```python
from build123d import *

# Parameters (mm, degrees)
SKETCH_1_R          = 13
EXTRUDE_1_DEPTH     = 4
SKETCH_2_R          = 6
CUT_EXTRUDE_1_DEPTH = 4
CUT_EXTRUDE_START   = -0.8
SKETCH_3_R          = 13
SKETCH_3_R_2        = 12
CUT_EXTRUDE_2_DEPTH = 0.4
CUT_EXTRUDE_START_2 = -3.2
SKETCH_3_3_R        = 13
SKETCH_3_3_R_2      = 12
CUT_EXTRUDE_3_DEPTH = 0.4


with BuildPart() as part:
    # Sketch 1 → Extrude 1 (new body)
    with BuildSketch(Plane(origin=(0, 0, 0), x_dir=(1, 0, 0), z_dir=(0, 1, 0))):
        Circle(SKETCH_1_R)
    extrude(amount=EXTRUDE_1_DEPTH)

    # Sketch 2 → Cut-Extrude 1 (cut)
    with BuildSketch(Plane.XZ):
        Circle(SKETCH_2_R)
    extrude(amount=-CUT_EXTRUDE_1_DEPTH, mode=Mode.SUBTRACT)

    # Sketch 3 → Cut-Extrude 2 (cut)
    with BuildSketch(Plane.XZ.offset(CUT_EXTRUDE_START)):
        Circle(SKETCH_3_R)
        Circle(SKETCH_3_R_2, mode=Mode.SUBTRACT)
    extrude(amount=-CUT_EXTRUDE_2_DEPTH, mode=Mode.SUBTRACT)

    # Sketch 3_3 → Cut-Extrude 3 (cut)
    with BuildSketch(Plane.XZ.offset(CUT_EXTRUDE_START_2)):
        Circle(SKETCH_3_3_R)
        Circle(SKETCH_3_3_R_2, mode=Mode.SUBTRACT)
    extrude(amount=CUT_EXTRUDE_3_DEPTH, mode=Mode.SUBTRACT)


solid = part.part
```
The model under review builds one solid part; all positions refer to its coordinate system, in mm. A direction names the side the tool comes from. Round coordinates to 2 decimals unless told otherwise and drop trailing zeros. Loops run counter-clockwise (first coordinate to the right, second up) from the corner with the lowest first, then second, coordinate; pieces in that order, holes last.
Item 1: Take a section at B-B (x = 0). Write out the cut boundary in (y, z), then the cut area to 3 significant figures.
Determined:
outline: (0, -13) - (0.8, -13) - (0.8, -12) - (1.2, -12) - (1.2, -13) - (2.8, -13) - (2.8, -12) - (3.2, -12) - (3.2, -13) - (4, -13) - (4, -6) - (0, -6) - close; (0, 6) - (4, 6) - (4, 13) - (3.2, 13) - (3.2, 12) - (2.8, 12) - (2.8, 13) - (1.2, 13) - (1.2, 12) - (0.8, 12) - (0.8, 13) - (0, 13) - close
area: 54.4 mm2
Item 2: Take a section at A-A (z = 0). Write out the cut boundary in (x, y).
Determined:
outline: (-13, 0) - (-6, 0) - (-6, 4) - (-13, 4) - (-13, 3.2) - (-12, 3.2) - (-12, 2.8) - (-13, 2.8) - (-13, 1.2) - (-12, 1.2) - (-12, 0.8) - (-13, 0.8) - close; (6, 0) - (13, 0) - (13, 0.8) - (12, 0.8) - (12, 1.2) - (13, 1.2) - (13, 2.8) - (12, 2.8) - (12, 3.2) - (13, 3.2) - (13, 4) - (6, 4) - close
Item 3: For faces 1 (the face through (6, 4, 3)), 2 (the face through (9, 0.8, -9)), list the 3-axis set-ups (+Z, -Z, +X, -X, +Y, -Y) from which the entire face can be reached by the end or side of a thin tool; tool diameter is ignored.
Determined:
face 1: +Z, -Z, +X, -X, +Y
face 2: none
Item 4: Take a section at D-D (x = -7.75). Write out the cut boundary in (y, z).
Determined:
outline: (0, -10.44) - (0.8, -10.44) - (0.8, -9.16) - (1.2, -9.16) - (1.2, -10.44) - (2.8, -10.44) - (2.8, -9.16) - (3.2, -9.16) - (3.2, -10.44) - (4, -10.44) - (4, 10.44) - (3.2, 10.44) - (3.2, 9.16) - (2.8, 9.16) - (2.8, 10.44) - (1.2, 10.44) - (1.2, 9.16) - (0.8, 9.16) - (0.8, 10.44) - (0, 10.44) - close
Item 5: Clearance check with a flat-ended pin moving along its axis: pin 1 Ø1 at (y, z) = (2.5, -8) entering from +X. State where the tip first meets the part, or that it passes through.
Determined:
pin 1: stops at x = 10.62
Item 6: Take a section at C-C (y = 1.8). Write out the cut boundary in (x, z).
Determined:
outline: circle Ø26 at (0, 0); hole circle Ø12 at (0, 0)
Item 7: For line 1 (Y direction, x = 11, z = -6.5); line 2 (X direction, y = 1.6, z = -0.25); line 3 (Z direction, x = 0, y = 1.05), list the stretches that pass through material, from the lowest coordinate up.
Determined:
line 1: y = 0 to 0.8, 1.2 to 2.8, 3.2 to 4
line 2: x = -13 to -5.99, 5.99 to 13
line 3: z = -12 to -6, 6 to 12
Item 8: Mouldability with a two-part tool opening along X and no side actions: class faces 3 (the face through (9, 3.2, -9)), 4 (the face through (-6, 2, 0)), 5 (the face through (-11.99, 3, 0.53)) as released by +X, released by -X, zero draft, split by the parting line, or undercut.
Determined:
face 3: zero draft
face 4: undercut
face 5: split by the parting line
